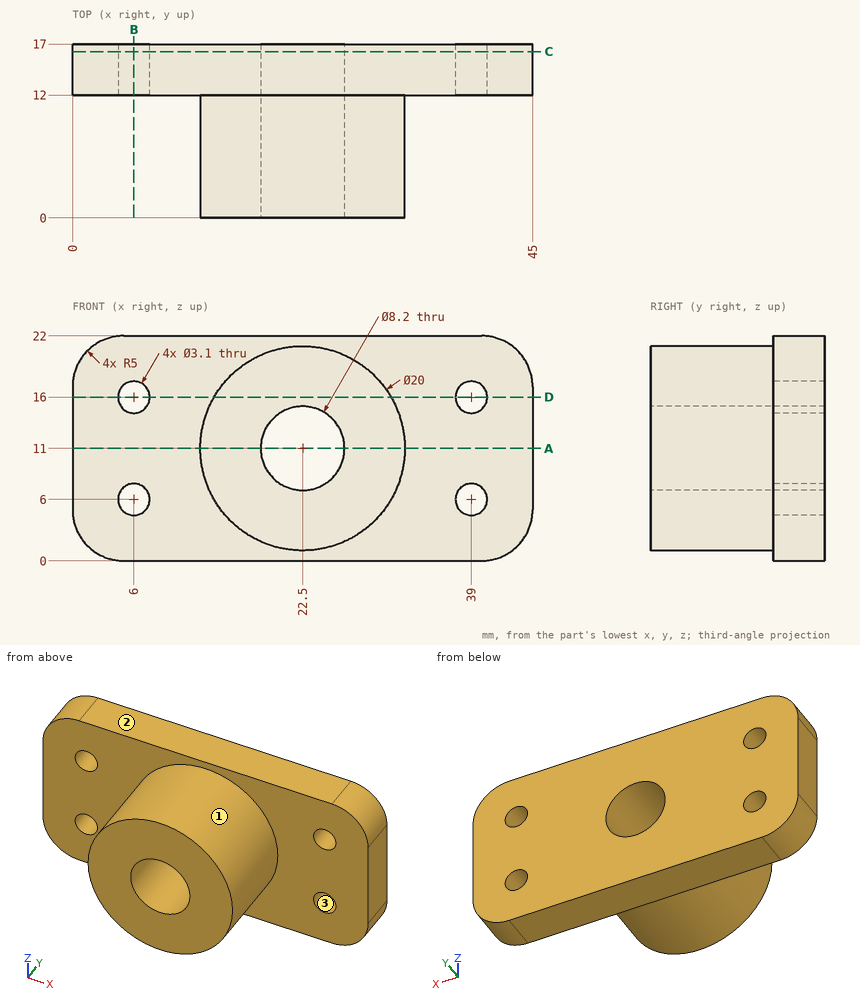
Geometry check sheet. Reference: drawing and pictorial views, mm from the part's lowest x, y, z. Round coordinates to 2 decimals unless told otherwise and drop trailing zeros. Loops run counter-clockwise (first coordinate to the right, second up) from the corner with the lowest first, then second, coordinate; pieces in that order, holes last. Notation, with made-up numbers: (-36.75, 84.25) - (3.25, 84.25) arc R18 ccw to (3.25, 113.25) - close; hole circle Ø3 at (61.5, 55). An arc over 180 degrees is marked (long way). Use a Markdown table: item, result. Add a question column.
1. Release check for a two-part mould opening along X. For the marked faces 1, 2 and 3 record: released by +X, released by -X, zero draft, split by the parting line, or undercut.
2. Section check C-C, the plane y = 16.25. Record the boundary of the cut face in (x, z), plus the area to 3 significant figures.
3. Section check B-B, the plane x = 6. Record the boundary of the cut face in (y, z).
4. Thickness scan on probe 1 along Z at (x, y) = (6, 16.05); probe 2 along Z at (x, y) = (22.5, 13); probe 3 along Y at (x, z) = (2.5, 7). Record the ranges inside material, lowest first. Write a range as [from, to].
5. Gauge pin test, flat ends, axial feed: pin 1 (2 mm diameter, centred on x = 19.5, y = 9.5, fed in from -Z); pin 2 (3 mm diameter, centred on y = 5, z = 13.5, fed in from +X); pin 3 (2.5 mm diameter, centred on x = 39, z = 16, fed in from -Y); pin 4 (1 mm diameter, centred on y = 2.5, z = 16, fed in from +X). Record the tip position at first contact, or that the pin passes through.
6. Section check D-D, the plane z = 16. Record the boundary of the cut face in (x, y), plus the area to 3 significant figures.
7. Section check A-A, the plane z = 11. Record the boundary of the cut face in (x, y), plus the area to 3 significant figures.
Checks:
| question | item | result |
|---|---|---|
| 1 | face 1 | split by the parting line |
| 1 | face 2 | zero draft |
| 1 | face 3 | undercut |
| 2 | outline | (0, 5) arc R5 ccw to (5, 0) - (40, 0) arc R5 ccw to (45, 5) - (45, 17) arc R5 ccw to (40, 22) - (5, 22) arc R5 ccw to (0, 17) - close; hole circle Ø3.1 at (6, 6); hole circle Ø3.1 at (6, 16); hole circle Ø8.2 at (22.5, 11); hole circle Ø3.1 at (39, 6); hole circle Ø3.1 at (39, 16) |
| 2 | area | 886 mm^2 |
| 3 | outline | (12, 0) - (17, 0) - (17, 4.45) - (12, 4.45) - close; (12, 7.55) - (17, 7.55) - (17, 14.45) - (12, 14.45) - close; (12, 17.55) - (17, 17.55) - (17, 22) - (12, 22) - close |
| 4 | probe 1 | z = [0, 4.45], [7.55, 14.45], [17.55, 22] |
| 4 | probe 2 | z = [0, 6.9], [15.1, 22] |
| 4 | probe 3 | y = [12, 17] |
| 5 | pin 1 | stops at z = 1.2 |
| 5 | pin 2 | stops at x = 32.45 |
| 5 | pin 3 | passes through |
| 5 | pin 4 | stops at x = 31.43 |
| 6 | outline | (0, 12) - (4.45, 12) - (4.45, 17) - (0, 17) - close; (7.55, 12) - (13.84, 12) - (13.84, 0) - (31.16, 0) - (31.16, 12) - (37.45, 12) - (37.45, 17) - (7.55, 17) - close; (40.55, 12) - (45, 12) - (45, 17) - (40.55, 17) - close |
| 6 | area | 402 mm^2 |
| 7 | outline | (0, 12) - (12.5, 12) - (12.5, 0) - (18.4, 0) - (18.4, 17) - (0, 17) - close; (26.6, 0) - (32.5, 0) - (32.5, 12) - (45, 12) - (45, 17) - (26.6, 17) - close |
| 7 | area | 326 mm^2 |
